```python
from build123d import *

# Parameters (mm, degrees)
BOSS_EXTRUDE1_DEPTH = 3
SKETCH2_W           = 4.5
SKETCH2_H           = 15
BOSS_EXTRUDE2_DEPTH = 15
CUT_EXTRUDE1_REACH  = 36.599
SKETCH3_R           = 1.7
FILLET1_R           = 7.5


with BuildPart() as part:
    # Sketch1 → Boss-Extrude1 (new body)
    with BuildSketch(Plane(origin=(0, 0, 0), x_dir=(1, 0, 0), z_dir=(0, 1, 0))):
        with BuildLine():
            Line((-6.25, -7.5), (-15.518088002, -14.494783398))
            ThreePointArc((-15.518088002, -14.494783398), (-16.255216602, -19.768088002), (-10.981911998, -20.505216602))
            Line((-10.981911998, -20.505216602), (6.25, -7.5))
            Line((6.25, -7.5), (6.25, 7.5))
            Line((6.25, 7.5), (-6.25, 7.5))
            Line((-6.25, 7.5), (-6.25, -7.5))
        make_face()
    extrude(amount=BOSS_EXTRUDE1_DEPTH)

    # Sketch2 → Boss-Extrude2 (add)
    with BuildSketch(Plane(origin=(0, 3, 0), x_dir=(1, 0, 0), z_dir=(0, 1, 0))):
        with Locations((1.25, 0)):
            Rectangle(SKETCH2_W, SKETCH2_H)
    extrude(amount=BOSS_EXTRUDE2_DEPTH)

    # Sketch3 → Cut-Extrude1 (cut, up to next)
    with BuildSketch(Plane(origin=(3.5, 0, 0), x_dir=(0, 0, -1), z_dir=(1, 0, 0)), mode=Mode.PRIVATE) as cut_extrude1_sk1:
        with Locations((0, 10.5)):
            Circle(SKETCH3_R)
    cut_extrude1_tool1 = extrude(cut_extrude1_sk1.sketch, amount=-CUT_EXTRUDE1_REACH, mode=Mode.PRIVATE) & part.part
    add(cut_extrude1_tool1.solids().sort_by_distance((3.5, 10.5, 0))[0], mode=Mode.SUBTRACT)

    # Fillet1
    fillet1_edges = [part.edges().sort_by_distance(p)[0] for p in [
        (1.25, 18, -7.5),
        (1.25, 18, 7.5),
    ]]
    fillet(fillet1_edges, radius=FILLET1_R - 0.0001)  # a hair under: the kernel refuses the full size


solid = part.part
```
The listing builds one solid part. Answer for the finished solid, in the listing's coordinates (mm). A direction names the side the tool comes from. Coordinates: 2 decimals unless noted, no trailing zeros. Write each loop counter-clockwise with the first axis right and the second up, starting at its lowest first coordinate (ties: lowest second). Pieces come first, ordered by that corner, then holes. Notation, with made-up numbers: (-39, -10.75) - (-25, -10.75) arc R16 cw to (-25, 16.25) - close; hole circle Ø5 at (36, 38.5). An arc over 180 degrees is marked (long way). One line per item, written item: value.
1) A tool of negligible diameter and unlimited length cuts with its end or side. For faces 4 (the flat face through (-6.25, 1, 0)), 5 (the flat face through (3.5, 10, 2)), 6 (the flat face through (-3, 0, 7)), 7 (the flat face through (-1, 10, 2)), 8 (the flat face through (1, 7, 7.5)), from which of +Z, -Z, +X, -X, +Y, -Y can it reach the whole face along a straight path? Write none if from no direction.
Geometry check:
face 4: -Z, -X, +Y, -Y
face 5: +Z, -Z, +X, +Y
face 6: +Z, -Z, +X, -X, -Y
face 7: +Z, -Z, -X, +Y
face 8: +Z, +X, -X, +Y
2) Find section C-C (z = -0.5). Give the vertices of the cut face in (x, y).
Geometry check:
outline: (-6.25, 0) - (6.25, 0) - (6.25, 3) - (3.5, 3) - (3.5, 8.88) - (-1, 8.88) - (-1, 3) - (-6.25, 3) - close; (-1, 12.12) - (3.5, 12.12) - (3.5, 17.98) - (-1, 17.98) - close
3) Each of these flat-tipped pins is pushed along its axis until it touches: pin 1 Ø4.5 at (y, z) = (14, -2) entering from -X; pin 2 Ø4 at (y, z) = (10.5, 0) entering from +X; pin 3 Ø2.5 at (y, z) = (2, -1.5) entering from -X. Where does it stop, or does it pass through?
Geometry check:
pin 1: stops at x = -1
pin 2: stops at x = 3.5
pin 3: stops at x = -6.25
4) Consider line 1 along Y through (x, z) = (1.2, 0); line 2 along X through (y, z) = (14.5, -3); line 3 along Z through (x, y) = (1, 5.25). Determine where each line is inside the solid, lowest interval first. Write a range as from..to.
Geometry check:
line 1: y = 0..8.8, 12.2..18
line 2: x = -1..3.5
line 3: z = -7.5..7.5
5) Find section D-D (y = 8.25). Give the vertices of the cut face in (x, z).
Geometry check:
outline: (-1, -7.5) - (3.5, -7.5) - (3.5, 7.5) - (-1, 7.5) - close
6) Find section A-A (y = 11.5). Give the vertices of the cut face in (x, z).
Geometry check:
outline: (-1, -7.43) - (3.5, -7.43) - (3.5, -1.37) - (-1, -1.37) - close; (-1, 1.37) - (3.5, 1.37) - (3.5, 7.43) - (-1, 7.43) - close
7) For a pull along Z with two mould halves and no side action, classify faces 1 (the cylindrical face through (-16.304, 1.479, 19.701)), 2 (the cylindrical face through (1.281, 12.186, 0.221)), 3 (the cylindrical face through (1.281, 15.745, -5.361)) as pulls with the +Z half, pulls with the -Z half, needs draft (parallel to the pull), parting line crosses it, or undercut.
Geometry check:
face 1: parting line crosses it
face 2: undercut
face 3: pulls with the -Z half
